Verification items for the finished model (mm, model axes). Face numbers are marked on the shaded views. A direction names the side the tool comes from. Round coordinates to 2 decimals unless told otherwise and drop trailing zeros. Loops run counter-clockwise (first coordinate to the right, second up) from the corner with the lowest first, then second, coordinate; pieces in that order, holes last. Notation, with made-up numbers: M 32,52.5 L 50,52.5 A24 cw 50,74.5 Z; hole C 54,-20.75 d7. An arc over 180 degrees is marked long. Write item = value, one per line. Start each with the question number.
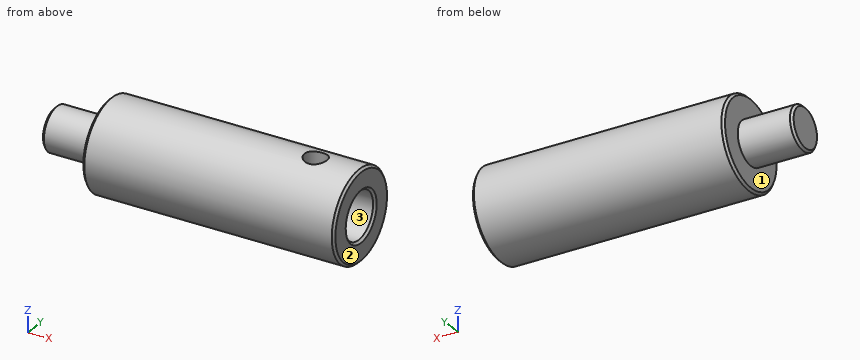
Autodesk Inventor part; units mm, degrees
ref_plane "Work Plane1" through (0, 0, 5) normal (0, 0, 1) x (1, 0, 0)
ref_plane "YZ Plane" through (0, 0, 0) normal (1, 0, 0) x (0, 1, 0)
ref_plane "XZ Plane" through (0, 0, 0) normal (0, 1, 0) x (-1, 0, 0)
sketch "Sketch2" plane through (0, 0, 0) normal (0, 1, 0) x (-1, 0, 0)
  line L0 (0.25, 5) -> (27.5, 5)
  line L1 (27.75, 4.75) -> (27.75, 2.4)
  line L2 (27.75, 2.4) -> (33.5, 2.4)
  line L3 (33.75, 2.15) -> (33.75, 0)
  line L4 (9.75, 2.6) -> (0.25, 2.6)
  line L5 (0, 2.85) -> (0, 4.75)
  line L6 (10, 2.35) -> (10, 0)
  line L7 (33.75, 2.15) -> (33.5, 2.4)
  line L8 (27.75, 4.75) -> (27.5, 5)
  line L9 (0.25, 5) -> (0, 4.75)
  line L10 (0, 2.85) -> (0.25, 2.6)
  line L11 (9.75, 2.6) -> (10, 2.35)
  line L12 (33.75, 0) -> (10, 0)
  point P0 (0, 0)
  point P1 (0, 5)
  point P2 (27.75, 5)
  point P3 (33.75, 2.4)
  point P4 (10, 2.6)
  point P5 (0, 2.6)
  dimension "d1" = 27.75
  dimension "d2" = 2.6
  dimension "d3" = 6
  dimension "d4" = 5
  dimension "d5" = 0.25
  dimension "d6" = 0.25
  dimension "d7" = 0.25
  dimension "d8" = 0.25
  dimension "d9" = 0.25
  dimension "d10" = 0.25
  dimension "d11" = 0.25
  dimension "d12" = 0.25
  dimension "d13" = 0.25
  dimension "d14" = 0.25
revolve "Revolution1" add sketch "Sketch2" angle 360 about axis through (-33.75, 0, 0) along (1, 0, 0)
ref_plane "Work Plane1" through (0, 0, 5) normal (0, 0, 1) x (1, 0, 0)
sketch "Sketch3" plane through (0, 0, 5) normal (0, 0, 1) x (1, 0, 0)
  circle A0 centre (-5, 0) radius 1.25
  point P0 (0, 0)
  dimension "d17" = 2.5
extrude "Extrusion1" cut sketch "Sketch3" against normal blind 5
thread "Thread1"
properties part number "ParrallelShaft"
1. Gauge pin test, flat ends, axial feed: P1, Ø1.5, axis at x = -14.5, y = -3, coming from the +Z side; P2, Ø1.5, axis at x = -5, y = 0, coming from the +Z side; P3, Ø2, axis at x = -8.5, y = 4, coming from the +Z side. Record the tip position at first contact, or that the pin passes through.
2. Section check D-D, the plane x = -5. Enter the section's corners in (y, z).
3. Thickness scan on line 1 (Y direction, x = -3.5, z = 0); line 2 (X direction, y = 0, z = 3.1). Record the ranges inside material, lowest first.
4. Section check C-C, the plane z = 0. Enter the section's corners in (x, y), and give its area (3 significant figures).
5. Section check B-B, the plane x = -9. Enter the section's corners in (y, z).
6. Tool access check on the marked faces 1, 2 and 3. Record the directions out of +Z, -Z, +X, -X, +Y, -Y that give a thin tool (end or side, any length) a straight path to the whole face; none if there is none.
7. Section check A-A, the plane y = 0. Enter the section's corners in (x, z), and give its area (3 significant figures).
Computed values:
q1.P1 = 4.47
q1.P2 = -2.49
q1.P3 = 4
q2.outline = M -1.25,2.28 L -1.25,4.84 A5 ccw long 1.25,4.84 L 1.25,2.28 A2.6 cw long Z
q3.line_1 = -5 to -2.6, 2.6 to 5
q3.line_2 = -27.75 to -6.25, -3.75 to 0
q4.outline = M -33.75,-2.15 L -33.5,-2.4 L -27.75,-2.4 L -27.75,-4.75 L -27.5,-5 L -0.25,-5 L 0,-4.75 L 0,-2.85 L -0.25,-2.6 L -9.75,-2.6 L -10,-2.35 L -10,2.35 L -9.75,2.6 L -0.25,2.6 L 0,2.85 L 0,4.75 L -0.25,5 L -27.5,5 L -27.75,4.75 L -27.75,2.4 L -33.5,2.4 L -33.75,2.15 Z
q4.area = 254 mm2
q5.outline = C 0,0 d10; hole C 0,0 d5.2
q6.face_1 = -X
q6.face_2 = +Z, -Z, +X, +Y, -Y
q6.face_3 = +X
q7.outline = M -33.75,-2.15 L -33.5,-2.4 L -27.75,-2.4 L -27.75,-4.75 L -27.5,-5 L -0.25,-5 L 0,-4.75 L 0,-2.85 L -0.25,-2.6 L -9.75,-2.6 L -10,-2.35 L -10,2.35 L -9.75,2.6 L -6.25,2.6 L -6.25,5 L -27.5,5 L -27.75,4.75 L -27.75,2.4 L -33.5,2.4 L -33.75,2.15 Z; M -3.75,2.6 L -0.25,2.6 L 0,2.85 L 0,4.75 L -0.25,5 L -3.75,5 Z
q7.area = 248 mm2
